```python
from build123d import *

# Parameters (mm, degrees)
BOX012_W               = 9.5
BOX012_H               = 900
BOX012_DEPTH           = 40
CYLINDER004_R          = 20
CYLINDER004_DEPTH      = 9.5
CYLINDER003_R          = 20
CYLINDER003_DEPTH      = 9.5
FUSION_PITCH_ANGLE     = 90
FUSION_PLACEMENT_ANGLE = -90
BOX011_W               = 1010
BOX011_H               = 5
BOX011_DEPTH           = 200
BOX010_W               = 1010
BOX010_H               = 5
BOX010_DEPTH           = 200
BOX_W                  = 1000
BOX_H                  = 500
BOX_DEPTH              = 200
THICKNESS_T            = 10


with BuildPart() as cube002:
    # Box012 → Box012 (new body)
    with BuildSketch(Plane(origin=(-8, 55, 119), x_dir=(1, 0, 0), z_dir=(0, 0, 1))):
        with Locations((4.75, 450)):
            Rectangle(BOX012_W, BOX012_H)
    extrude(amount=BOX012_DEPTH)


with BuildPart() as cylinder004:
    # Cylinder004 → Cylinder004 (new body)
    with BuildSketch(Plane(origin=(1.5, 955, 139), x_dir=(0, 0, 1), z_dir=(-1, 0, 0))):
        Circle(CYLINDER004_R)
    extrude(amount=CYLINDER004_DEPTH)


with BuildPart() as windows:
    # Cylinder003 → Cylinder003 (new body)
    with BuildSketch(Plane(origin=(1.5, 55, 139), x_dir=(0, 0, 1), z_dir=(-1, 0, 0))):
        Circle(CYLINDER003_R)
    extrude(amount=CYLINDER003_DEPTH)

    # Fusion: union Cube002, Cylinder004
    add(cube002.part)
    add(cylinder004.part)


with BuildPart() as windows_1:
    # Fusion pitch: moved
    add(windows.part.rotate(Axis((0, 0, 0), (0, 1, 0)), FUSION_PITCH_ANGLE))


with BuildPart() as windows_2:
    # Fusion placement: moved
    add(windows_1.part.moved(Location((0, 337.5, -10))).rotate(Axis((0, 337.5, -10), (0, 0, 1)), FUSION_PLACEMENT_ANGLE))


with BuildPart() as supportrail002:
    # Box011 → Box011 (new body)
    with BuildSketch(Plane(origin=(-5.7935, 85.5, 65), x_dir=(1, 0, 0), z_dir=(0, 0, 1))):
        with Locations((505, 2.5)):
            Rectangle(BOX011_W, BOX011_H)
    extrude(amount=BOX011_DEPTH)


with BuildPart() as supportrail001:
    # Box010 → Box010 (new body)
    with BuildSketch(Plane(origin=(-5.7935, 454, 65), x_dir=(1, 0, 0), z_dir=(0, 0, 1))):
        with Locations((505, 2.5)):
            Rectangle(BOX010_W, BOX010_H)
    extrude(amount=BOX010_DEPTH)


with BuildPart() as obj1:
    # Box → Box (new body)
    with BuildSketch(Plane.XY):
        with Locations((500, 250)):
            Rectangle(BOX_W, BOX_H)
    extrude(amount=BOX_DEPTH)

    # Thickness
    thickness_openings = [obj1.faces().sort_by_distance(p)[0] for p in [
        (500, 250, 200),
    ]]
    offset(amount=THICKNESS_T, openings=thickness_openings)

    # Cut: cut SupportRail001
    add(supportrail001.part, mode=Mode.SUBTRACT)

    # Cut001: cut SupportRail002
    add(supportrail002.part, mode=Mode.SUBTRACT)

    # Cut002: cut Windows
    add(windows_2.part, mode=Mode.SUBTRACT)


solid = obj1.part
```
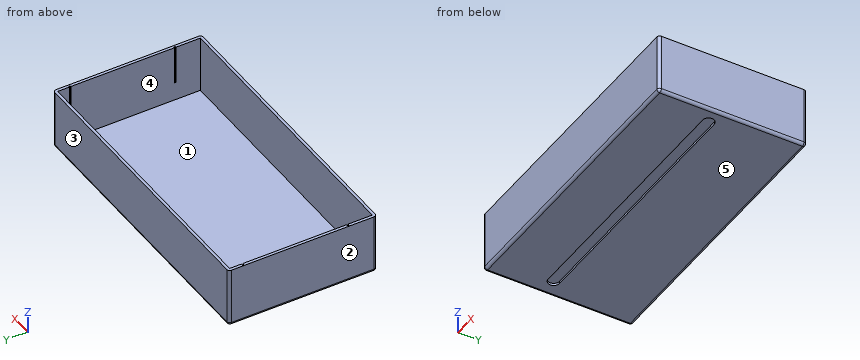
Check sheet for the modelled part. Datum: model origin and axes. Units: mm. Face numbers are marked on the shaded views. A direction names the side the tool comes from. Round coordinates to 2 decimals unless told otherwise and drop trailing zeros. Loops run counter-clockwise (first coordinate to the right, second up) from the corner with the lowest first, then second, coordinate; pieces in that order, holes last. Notation, with made-up numbers: M -8.5,71 L 9.5,71 A20 ccw 9.5,97 Z; hole C 52.25,49 d2. An arc over 180 degrees is marked long. Answer as a JSON object with one key per item and string values.
1. Gauge pin test, flat ends, axial feed: P1, Ø3, axis at x = -2, z = 154.5, coming from the +Y side; P2, Ø3.5, axis at x = 1001.5, y = 88.5, coming from the +Z side; P3, Ø4.5, axis at x = 1003, z = 123.5, coming from the -Y side. Record the tip position at first contact, or that the pin passes through.
Reply:
{"P1": "stops at y = 509.99", "P2": "stops at z = 65", "P3": "stops at y = -9.97"}
2. Section check C-C (x = 354). Record the boundary of the cut face in (y, z), plus the area to 3 significant figures.
Reply:
{"outline": "M -10,0 A10 ccw 0,-10 L 178.5,-10 L 178.5,-2 L 218.5,-2 L 218.5,-10 L 500,-10 A10 ccw 510,0 L 510,200 L 500,200 L 500,0 L 0,0 L 0,200 L -10,200 Z", "area": "8,840 mm²"}
3. Section check A-A (z = 135). Record the boundary of the cut face in (x, y).
Reply:
{"outline": "M -10,0 A10 ccw 0,-10 L 1000,-10 A10 ccw 1010,0 L 1010,500 A10 ccw 1000,510 L 0,510 A10 ccw -10,500 Z; hole M -5.79,85.5 L 0,85.5 L 0,0 L 1000,0 L 1000,85.5 L 1004.21,85.5 L 1004.21,90.5 L 1000,90.5 L 1000,454 L 1004.21,454 L 1004.21,459 L 1000,459 L 1000,500 L 0,500 L 0,459 L -5.79,459 L -5.79,454 L 0,454 L 0,90.5 L -5.79,90.5 Z"}
4. Section check B-B (y = 265.5). Record the boundary of the cut face in (x, z), plus the area to 3 significant figures.
Reply:
{"outline": "M -10,0 A10 ccw 0,-10 L 1000,-10 A10 ccw 1010,0 L 1010,200 L 1000,200 L 1000,0 L 0,0 L 0,200 L -10,200 Z", "area": "14,200 mm²"}
5. Mould release check, pull along Y, two halves, no side actions. Record for the marked faces 1, 2 and 3: pulls with the +Y half, pulls with the -Y half, needs draft (parallel to the pull), parting line crosses it, or undercut.
Reply:
{"face 1": "undercut", "face 2": "needs draft", "face 3": "pulls with the +Y half"}
6. Scan lines: line 1 (X direction, y = 341, z = 162); line 2 (Y direction, x = 297.5, z = 18.5); line 3 (Z direction, x = 820, y = 80.5). Record each from-to range of solid material in increasing order.
Reply:
{"line 1": "x = -10 to 0, 1000 to 1010", "line 2": "y = -10 to 0, 500 to 510", "line 3": "z = -10 to 0"}
7. Access from +Z, -Z, +X, -X, +Y, -Y to the whole of each face (thin tool, end or side, straight path). Record for the marked faces 4 and 5.
Reply:
{"face 4": "+Z", "face 5": "-Z, +X, -X, +Y, -Y"}
8. Section check D-D (z = 36). Record the boundary of the cut face in (x, y).
Reply:
{"outline": "M -10,0 A10 ccw 0,-10 L 1000,-10 A10 ccw 1010,0 L 1010,500 A10 ccw 1000,510 L 0,510 A10 ccw -10,500 Z; hole M 0,0 L 1000,0 L 1000,500 L 0,500 Z"}
